from build123d import *

# Parameters (mm, degrees)
F0_W     = 150
F0_H     = 86
F0_R     = 1.9812
F1_DEPTH = 180
F2_R     = 65
F3_DEPTH = 80
F4_W     = 13.712838
F4_H     = 20.182729
F5_DEPTH = 12.7


with BuildPart() as f1:
    # F0 (on Front) → F1 (new body)
    with BuildSketch(Plane.XZ):
        Rectangle(F0_W, F0_H)
        with Locations((-69, -27)):
            Circle(F0_R, mode=Mode.SUBTRACT)
        with Locations((69, -37)):
            Circle(F0_R, mode=Mode.SUBTRACT)
        with Locations((-69, 37)):
            Circle(F0_R, mode=Mode.SUBTRACT)
        with Locations((69, 37)):
            Circle(F0_R, mode=Mode.SUBTRACT)
    extrude(amount=F1_DEPTH)

    # F2 (on face) → F3 (cut)
    with BuildSketch(Plane.XY.offset(43)):
        with Locations((0, -92)):
            Circle(F2_R)
    extrude(amount=-F3_DEPTH, mode=Mode.SUBTRACT)

    # F4 (on face) → F5 (join)
    with BuildSketch(Plane.XZ.offset(180)):
        with Locations((47.160495, -10.091364)):
            Rectangle(F4_W, F4_H)
    extrude(amount=F5_DEPTH)


solid = f1.part
Could you check a few things on this model? Use its own coordinates, in mm. A direction names the side the tool comes from. Coordinates: 2 decimals unless noted, no trailing zeros. Order: outer loops, then holes, each group sorted by start corner. A loop starts at its lowest first (then second) coordinate and runs counter-clockwise, first axis right, second up. Notation, with made-up numbers: (58, 20) -> (105, 20) arc R29 cw to (105, 50) -> close; hole circle Ø5 at (54.25, 18.25). An arc over 180 degrees is marked (long way). One line per item, written item: value. Start each with the question number.
1) If I drill on L1, parallel to Z at x = -69, y = -95; L2, parallel to Z at x = 69, y = -138.5; L3, parallel to Z at x = -31, y = -99.5, over which ranges is the centre line in solid material (lowest first)? Write a range as [from, to].
2) We'd pull the mould along X, two halves only. Please class faces 1 (the flat face through (47, -186, 0)), 2 (the flat face through (40.304, -186, -10)), 3 (the cylindrical face through (-67.11, -88.74, -26.4)): +X half, -X half, draft (parallel to the pull), parting line (faces both ways), or undercut.
3) Which directions (+Z, -Z, +X, -X, +Y, -Y) give clear straight access to the entire face, cutting with the end or side of a thin tool? Please do faces 4 (the flat face through (54.017, -186, -10)), 5 (the flat face through (47, -186, -20.183)), 6 (the cylindrical face through (62, -72.48, 3.56)).
4) Imagine slicing it at D-D on z = -12. List the corners of the cut face in (x, y) for me.
5) Imagine slicing it at B-B on y = -92. List the corners of the cut face in (x, z) for me, plus the area to 3 significant figures.
6) Imagine slicing it at A-A on z = 28. List the corners of the cut face in (x, y) for me, plus the area to 3 significant figures.
7) I'm going to push flat-ended pins straight in: pin 1 (6.5 mm diameter, centred on x = -69, z = 37, fed in from -Y); pin 2 (4 mm diameter, centred on y = -185.5, z = -14, fed in from +X); pin 3 (4 mm diameter, centred on x = 45.5, y = -183, fed in from +Z); pin 4 (3.5 mm diameter, centred on x = -69, z = -27, fed in from -Y). Where does each tip first touch, or does it pass through?
8) Imagine slicing it at C-C on x = 0. List the corners of the cut face in (y, z) for me, plus the area to 3 significant figures.
Answer list:
1. L1: z = [-43, -28.98], [-25.02, 35.02], [38.98, 43]
1. L2: z = [-43, -38.98], [-35.02, 35.02], [38.98, 43]
1. L3: z = [-43, -37]
2. face 1: draft
2. face 2: -X half
2. face 3: undercut
3. face 4: +Z, -Z, +X, -Y
3. face 5: -Z, +X, -X, -Y
3. face 6: +Z
4. outline: (-75, -180) -> (40.3, -180) -> (40.3, -192.7) -> (54.02, -192.7) -> (54.02, -180) -> (75, -180) -> (75, 0) -> (-75, 0) -> close; hole circle Ø130 at (0, -92)
5. outline: (-75, -43) -> (75, -43) -> (75, 43) -> (65, 43) -> (65, -37) -> (-65, -37) -> (-65, 43) -> (-75, 43) -> close; hole circle Ø3.96 at (-69, -27); hole circle Ø3.96 at (-69, 37); hole circle Ø3.96 at (69, -37); hole circle Ø3.96 at (69, 37)
5. area: 2,450 mm2
6. outline: (-75, -180) -> (75, -180) -> (75, 0) -> (-75, 0) -> close; hole circle Ø130 at (0, -92)
6. area: 13,700 mm2
7. pin 1: stops at y = -180
7. pin 2: stops at x = 54.02
7. pin 3: stops at z = 0
7. pin 4: passes through
8. outline: (-180, -43) -> (0, -43) -> (0, 43) -> (-27, 43) -> (-27, -37) -> (-157, -37) -> (-157, 43) -> (-180, 43) -> close
8. area: 5,080 mm2
